Verification items for the finished model (mm, model axes). Round coordinates to 2 decimals unless told otherwise and drop trailing zeros. Loops run counter-clockwise (first coordinate to the right, second up) from the corner with the lowest first, then second, coordinate; pieces in that order, holes last. Notation, with made-up numbers: M 52,74 L 58,74 A21 ccw 58,108 Z; hole C 61,-12 d3. An arc over 180 degrees is marked long. One line per item, written item: value.
from build123d import *

# Parameters (mm, degrees)
BOSS_EXTRUDE1_DEPTH = 2.5
FILLET1_R           = 1
CHAMFER1_SIZE       = 0.5


with BuildPart() as part:
    # Sketch1 → Boss-Extrude1 (new body)
    with BuildSketch(Plane(origin=(0, 0, 0), x_dir=(1, 0, 0), z_dir=(0, 1, 0))):
        with BuildLine():
            Line((-3.3, 0), (-3.3, -2))
            Line((-3.3, -2), (-6, -2))
            Line((-6, -2), (-6, 0))
            ThreePointArc((-6, 0), (-5.196152423, 3), (-3, 5.196152423))
            Line((-3, 5.196152423), (-3, 40.196152423))
            Line((-3, 40.196152423), (3, 40.196152423))
            Line((3, 40.196152423), (3, 5.196152423))
            ThreePointArc((3, 5.196152423), (5.196152423, 3), (6, 0))
            Line((6, 0), (6, -2))
            Line((6, -2), (3.3, -2))
            Line((3.3, -2), (3.3, 0))
            ThreePointArc((3.3, 0), (0, 3.3), (-3.3, 0))
        make_face()
    extrude(amount=BOSS_EXTRUDE1_DEPTH)

    # Fillet1
    fillet1_edges = [part.edges().sort_by_distance(p)[0] for p in [
        (-3.3, 1.25, 2),
        (-6, 1.25, 2),
        (-3, 1.25, -40.196152423),
        (3, 1.25, -40.196152423),
        (6, 1.25, 2),
        (3.3, 1.25, 2),
    ]]
    fillet(fillet1_edges, radius=FILLET1_R)

    # Chamfer1
    chamfer1_edges = [part.edges().sort_by_distance(p)[0] for p in [
        (-6, 0, 0.5),
        (-5.196152423, 0, -3),
        (3, 0, -22.196152423),
        (5.196152423, 0, -3),
        (3.3, 0, 0.5),
        (0, 0, -3.3),
        (5.196152423, 2.5, -3),
        (3, 2.5, -22.196152423),
        (-3, 0, -22.196152423),
        (-3, 2.5, -22.196152423),
        (-5.196152423, 2.5, -3),
        (-3.3, 0, 0.5),
        (-4.65, 0, 2),
        (0, 0, -40.196152423),
        (6, 0, 0.5),
        (4.65, 0, 2),
        (-6, 2.5, 0.5),
        (-5.707106781, 0, 1.707106781),
        (-3.592893219, 0, 1.707106781),
        (3.592893219, 0, 1.707106781),
        (5.707106781, 0, 1.707106781),
        (2.707106781, 0, -39.903259204),
        (-2.707106781, 0, -39.903259204),
        (0, 2.5, -40.196152423),
        (4.65, 2.5, 2),
        (6, 2.5, 0.5),
        (-4.65, 2.5, 2),
        (-3.3, 2.5, 0.5),
        (-5.707106781, 2.5, 1.707106781),
        (-3.592893219, 2.5, 1.707106781),
        (0, 2.5, -3.3),
        (3.592893219, 2.5, 1.707106781),
        (5.707106781, 2.5, 1.707106781),
        (2.707106781, 2.5, -39.903259204),
        (-2.707106781, 2.5, -39.903259204),
        (3.3, 2.5, 0.5),
    ]]
    chamfer(chamfer1_edges, length=CHAMFER1_SIZE)


solid = part.part
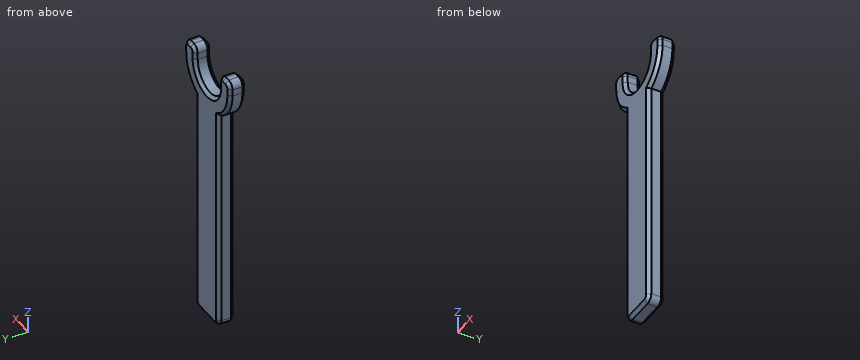
(1) Sectioned sample at C-C on z = -13. Enter the section's corners in (x, y).
Completed:
outline: M -3,0.5 L -2.5,0 L 2.5,0 L 3,0.5 L 3,2 L 2.5,2.5 L -2.5,2.5 L -3,2 Z
(2) Sectioned sample at B-B on x = 0. Enter the section's corners in (y, z), and give its area (3 significant figures).
Completed:
outline: M 0,-39.7 L 0.5,-40.2 L 2,-40.2 L 2.5,-39.7 L 2.5,-3.8 L 2,-3.3 L 0.5,-3.3 L 0,-3.8 Z
area: 91.7 mm^2
(3) Sectioned sample at A-A on y = 1.1. Enter the section's corners in (x, z), and give its area (3 significant figures).
Completed:
outline: M -6,0 A6 ccw -3,-5.2 L -3,-39.2 A1 ccw -2,-40.2 L 2,-40.2 A1 ccw 3,-39.2 L 3,-5.2 A6 ccw 6,0 L 6,1 A1 ccw 5,2 L 4.3,2 A1 ccw 3.3,1 L 3.3,0 A3.3 cw -3.3,0 L -3.3,1 A1 ccw -4.3,2 L -5,2 A1 ccw -6,1 Z
area: 256 mm^2
(4) Depth check by flat-ended pin: pin 1 Ø0.8 at (y, z) = (1, -22.5) entering from +X; pin 2 Ø4 at (x, z) = (-3, -13.5) entering from -Y; pin 3 Ø0.8 at (y, z) = (1, -15) entering from -X. Enter the tip coordinate at first touch or a pass-through.
Completed:
pin 1: stops at x = 3
pin 2: stops at y = 0
pin 3: stops at x = -3
(5) Thickness scan on L1, parallel to X at y = 1.2, z = -15; L2, parallel to X at y = 1.6, z = -3; L3, parallel to Z at x = 4.5, y = 2.15. Record the ranges inside material, lowest first. Write a range as from..to.
Completed:
L1: x = -3..3
L2: x = -5.2..-1.37, 1.37..5.2
L3: z = -3.74..1.85
